Can you work these out from the model? Positions are in its coordinate system, mm. Face numbers are marked on the shaded views. A direction names the side the tool comes from. Round coordinates to 2 decimals unless told otherwise and drop trailing zeros. Order: outer loops, then holes, each group sorted by start corner. A loop starts at its lowest first (then second) coordinate and runs counter-clockwise, first axis right, second up. Notation, with made-up numbers: (63, 50) -> (91, 50) arc R22 cw to (91, 59) -> close; hole circle Ø2 at (-28, -28.75). An arc over 180 degrees is marked (long way). One line per item, written item: value.
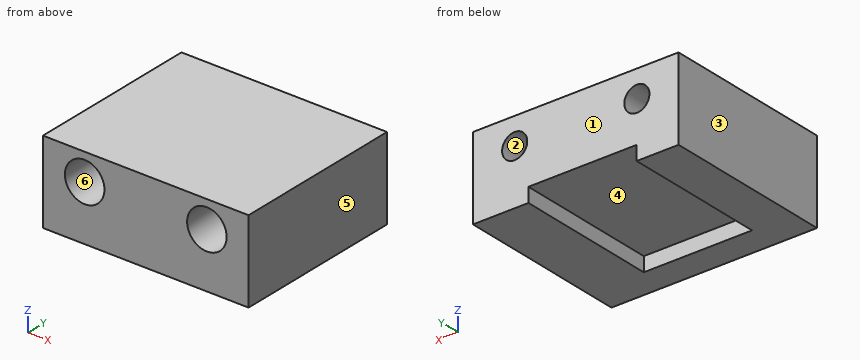
```python
from build123d import *

# Parameters (mm, degrees)
SKETCH018_R     = 1.75
PAD009_DEPTH    = 20
SKETCH019_W     = 28.6
SKETCH019_H     = 11.45
SKETCH019_R     = 1.75
PAD010_DEPTH    = 4
SKETCH020_R     = 2.75
POCKET009_DEPTH = 8


with BuildPart() as part:
    # Sketch018 (on Face21 of Binder005) → Pad009 (new body)
    with BuildSketch(Plane.XZ.offset(-32.95)):
        Polygon((-0.55022, 13.05), (28.04978, 13.05), (28.04978, 1.6), (20.338297, 1.6), (20.338297, 3.6), (5.278297, 3.6), (5.278297, 1.6), (-0.55022, 1.6), align=None)
        with Locations((5.24978, 9.3)):
            Circle(SKETCH018_R, mode=Mode.SUBTRACT)
        with Locations((22.24978, 9.3)):
            Circle(SKETCH018_R, mode=Mode.SUBTRACT)
    extrude(amount=PAD009_DEPTH)

    # Sketch019 (on Face12 of Pad009) → Pad010 (join)
    with BuildSketch(Plane.XZ.offset(-12.95)):
        with Locations((13.74978, 7.325)):
            Rectangle(SKETCH019_W, SKETCH019_H)
        with Locations((5.24978, 9.3)):
            Circle(SKETCH019_R, mode=Mode.SUBTRACT)
        with Locations((22.24978, 9.3)):
            Circle(SKETCH019_R, mode=Mode.SUBTRACT)
    extrude(amount=PAD010_DEPTH)

    # Sketch020 (on Face1 of Pad010) → Pocket009 (cut)
    with BuildSketch(Plane.XZ.offset(-8.95)):
        with Locations((22.24978, 9.3)):
            Circle(SKETCH020_R)
        with Locations((5.24978, 9.3)):
            Circle(SKETCH020_R)
    extrude(amount=-POCKET009_DEPTH, mode=Mode.SUBTRACT)


solid = part.part
```
Q1. I want a section at B-B on y = 16.25. List the corners of the cut face in (x, z) for me.
Answers below:
outline: (-0.55, 1.6) -> (5.28, 1.6) -> (5.28, 3.6) -> (20.34, 3.6) -> (20.34, 1.6) -> (28.05, 1.6) -> (28.05, 13.05) -> (-0.55, 13.05) -> close; hole circle Ø5.5 at (5.25, 9.3); hole circle Ø5.5 at (22.25, 9.3)
Q2. I want a section at D-D on y = 26.75. List the corners of the cut face in (x, z) for me.
Answers below:
outline: (-0.55, 1.6) -> (5.28, 1.6) -> (5.28, 3.6) -> (20.34, 3.6) -> (20.34, 1.6) -> (28.05, 1.6) -> (28.05, 13.05) -> (-0.55, 13.05) -> close; hole circle Ø3.5 at (5.25, 9.3); hole circle Ø3.5 at (22.25, 9.3)
Q3. We'd pull the mould along X, two halves only. Please class the marked faces 1, 2 and 3: released by +X, released by -X, zero draft, split by the parting line, or undercut.
Answers below:
face 1: zero draft
face 2: undercut
face 3: released by -X
Q4. Please list where these lines run through material, in increasing order: line 1 along X through (y, z) = (22.75, 9.3); line 2 along X through (y, z) = (23.25, 10.75); line 3 along X through (y, z) = (18.5, 2.5).
Answers below:
line 1: -0.55 to 3.5, 7 to 20.5, 24 to 28.05
line 2: -0.55 to 4.27, 6.23 to 21.27, 23.23 to 28.05
line 3: -0.55 to 5.28, 20.34 to 28.05
Q5. I want a section at C-C on z = 2.75. List the corners of the cut face in (x, y) for me.
Answers below:
outline: (-0.55, 8.95) -> (28.05, 8.95) -> (28.05, 32.95) -> (20.34, 32.95) -> (20.34, 12.95) -> (5.28, 12.95) -> (5.28, 32.95) -> (-0.55, 32.95) -> close
Q6. I want a section at A-A on z = 9.3. List the corners of the cut face in (x, y) for me.
Answers below:
outline: (-0.55, 8.95) -> (2.5, 8.95) -> (2.5, 16.95) -> (3.5, 16.95) -> (3.5, 32.95) -> (-0.55, 32.95) -> close; (7, 16.95) -> (8, 16.95) -> (8, 8.95) -> (19.5, 8.95) -> (19.5, 16.95) -> (20.5, 16.95) -> (20.5, 32.95) -> (7, 32.95) -> close; (24, 16.95) -> (25, 16.95) -> (25, 8.95) -> (28.05, 8.95) -> (28.05, 32.95) -> (24, 32.95) -> close
Q7. On a 3-axis mill with a long thin cutter (end or side, diameter ignored), from which of +Z, -Z, +X, -X, +Y, -Y can I reach the whole of each face in a straight line? I mean the marked faces 4, 5 and 6. Say none if no direction works.
Answers below:
face 4: -Z, +Y
face 5: +Z, -Z, +X, +Y, -Y
face 6: -Y
Q8. Will these pins go through, and if not, where does the flat tip stop? pin 1 Ø6 at (x, z) = (22.5, 8.5) entering from -Y; pin 2 Ø1.6 at (x, z) = (6.5, 8.5) entering from -Y.
Answers below:
pin 1: y = 8.95
pin 2: y = 16.95
